For this review, take the finished solid that the model builds, in its own axes (mm). Round coordinates to 2 decimals unless told otherwise and drop trailing zeros. Order: outer loops, then holes, each group sorted by start corner. A loop starts at its lowest first (then second) coordinate and runs counter-clockwise, first axis right, second up. Notation, with made-up numbers: (2.25, 31.5) -> (36.25, 31.5) arc R15 ccw to (36.25, 39.5) -> close; hole circle Ø5 at (42.5, 54). An arc over 180 degrees is marked (long way). Use a Markdown table: item, result. Add a question column.
1) Wall thickness on line 1 along Z through (x, y) = (-2, -10.5); line 2 along X through (y, z) = (6.25, 0.5); line 3 along Y through (x, z) = (-40, 3.75): over which ranges is each line inside the solid? List them lowest first. Write a range as [from, to].
2) Clearance check with flat-ended pins moving along their axes: P1, Ø1.5, axis at y = 8, z = 0.5, coming from the -X side; P2, Ø1.1, axis at y = -14.5, z = -0.5, coming from the +X side; P3, Ø0.5, axis at x = 13, y = -14.5, coming from the +Z side; P4, Ø6.5, axis at x = -22, z = 0.5, coming from the -Y side. State where each tip first meets the part, or that it passes through.
3) Consider section B-B (x = -285.5). State the section outline as (y, z) points, plus the area to 3 significant figures.
4) Consider section A-A (x = 14.5). State the section outline as (y, z) points.
```python
from build123d import *

# Parameters (mm, degrees)
SKETCH_W        = 100
SKETCH_H        = 30
PAD_DEPTH       = 5.5
FILLET_R        = 5
THICKNESS_T     = -1
PAD001_DEPTH    = 2
CHAMFER_SIZE    = 1
SKETCH002_R     = 3
HOLE_DEPTH      = 25
HOLE_TIPS_R     = 3
SKETCH003_R     = 0.75
SKETCH003_W     = 14
SKETCH003_H     = 6
POCKET_DEPTH    = 5
SKETCH004_R     = 3.25
PAD002_DEPTH    = 10
SKETCH005_R     = 2
PAD003_DEPTH    = 258.5
SKETCH006_R     = 2.5
PAD004_DEPTH    = 6
PAD005_DEPTH    = 18
PAD006_DEPTH    = 7.5
POCKET001_DEPTH = 7


with BuildPart() as part:
    # Sketch → Pad (new body, symmetric)
    with BuildSketch(Plane.XY):
        Rectangle(SKETCH_W, SKETCH_H)
    extrude(amount=PAD_DEPTH, both=True)

    # Fillet
    fillet_edges = [part.edges().sort_by_distance(p)[0] for p in [
        (-50, -15, 0),
        (-50, 15, 0),
        (50, 15, 0),
        (50, -15, 0),
    ]]
    fillet(fillet_edges, radius=FILLET_R)

    # Thickness
    thickness_openings = [part.faces().sort_by_distance(p)[0] for p in [
        (0, 0, -5.5),
    ]]
    offset(amount=THICKNESS_T, openings=thickness_openings)

    # Sketch001 (on Face10 of Thickness) → Pad001 (join)
    with BuildSketch(Plane(origin=(0, 0, -5.5), x_dir=(1, 0, 0), z_dir=(0, 0, -1))):
        with BuildLine():
            ThreePointArc((-45, 14), (-47.828427, 12.828427), (-49, 10))
            Line((-49, -10), (-49, 10))
            ThreePointArc((-49, -10), (-47.828427, -12.828427), (-45, -14))
            Line((45, -14), (-45, -14))
            ThreePointArc((45, -14), (47.828427, -12.828427), (49, -10))
            Line((49, 10), (49, -10))
            ThreePointArc((49, 10), (47.828427, 12.828427), (45, 14))
            Line((-45, 14), (45, 14))
        make_face()
    extrude(amount=-PAD001_DEPTH)

    # Chamfer
    chamfer_edges = [part.edges().sort_by_distance(p)[0] for p in [
        (0, -15, 5.5),
        (48.535534, -13.535534, 5.5),
        (50, 0, 5.5),
        (48.535534, 13.535534, 5.5),
        (0, 15, 5.5),
        (-48.535534, 13.535534, 5.5),
        (-50, 0, 5.5),
        (-48.535534, -13.535534, 5.5),
    ]]
    chamfer(chamfer_edges, length=CHAMFER_SIZE)

    # Sketch002 (on Face7 of Chamfer) → Hole (cut)
    with BuildSketch(Plane(origin=(-50, 0, 0), x_dir=(0, -1, 0), z_dir=(-1, 0, 0))):
        Circle(SKETCH002_R)
    extrude(amount=-HOLE_DEPTH, mode=Mode.SUBTRACT)

    # Hole tips → Hole tip 1 section 0
    with BuildSketch(Plane(origin=(-25, 0, 0), x_dir=(0, -1, 0), z_dir=(-1, 0, 0)), mode=Mode.PRIVATE) as hole_tip_1_s0:
        Circle(HOLE_TIPS_R)
    loft([hole_tip_1_s0.sketch, Vertex(-23.197418, 0, 0)], mode=Mode.SUBTRACT)

    # Sketch003 (on Face11 of Hole) → Pocket (cut)
    with BuildSketch(Plane.XZ.offset(15)):
        with Locations((-37.906574, 2.290524)):
            Circle(SKETCH003_R)
        with Locations((35.604452, 0)):
            Rectangle(SKETCH003_W, SKETCH003_H)
        with Locations((14.604452, 0)):
            Rectangle(SKETCH003_W, SKETCH003_H)
        with Locations((-6.395548, 0)):
            Rectangle(SKETCH003_W, SKETCH003_H)
        with Locations((-27.395548, 0)):
            Rectangle(SKETCH003_W, SKETCH003_H)
    extrude(amount=-POCKET_DEPTH, mode=Mode.SUBTRACT)

    # Sketch004 (on Face7 of Pocket) → Pad002 (join)
    with BuildSketch(Plane(origin=(-50, 0, 0), x_dir=(0, -1, 0), z_dir=(-1, 0, 0))):
        Circle(SKETCH004_R)
    extrude(amount=PAD002_DEPTH)

    # Sketch005 (on Face38 of Pad002) → Pad003 (join)
    with BuildSketch(Plane(origin=(-60, 0, 0), x_dir=(0, -1, 0), z_dir=(-1, 0, 0))):
        Circle(SKETCH005_R)
    extrude(amount=PAD003_DEPTH)

    # Sketch006 (on Face45 of Pad003) → Pad004 (join)
    with BuildSketch(Plane(origin=(-318.5, 0, 0), x_dir=(0, -1, 0), z_dir=(-1, 0, 0))):
        Circle(SKETCH006_R)
    extrude(amount=PAD004_DEPTH)

    # Sketch007 (on Face3 of Pad004) → Pad005 (join)
    with BuildSketch(Plane(origin=(-324.5, 0, 0), x_dir=(0, -1, 0), z_dir=(-1, 0, 0))):
        with BuildLine():
            ThreePointArc((-3, 2.5), (-5.5, 0), (-3, -2.5))
            Line((-3, -2.5), (3, -2.5))
            ThreePointArc((3, -2.5), (5.5, 0), (3, 2.5))
            Line((3, 2.5), (-3, 2.5))
        make_face()
    extrude(amount=PAD005_DEPTH)

    # Sketch008 (on Face11 of Pad005) → Pad006 (join)
    with BuildSketch(Plane(origin=(-342.5, 0, 0), x_dir=(0, -1, 0), z_dir=(-1, 0, 0))):
        with BuildLine():
            ThreePointArc((-3.25, 1.25), (-4.5, 0), (-3.25, -1.25))
            Line((-3.25, -1.25), (3.25, -1.25))
            ThreePointArc((3.25, -1.25), (4.5, 0), (3.25, 1.25))
            Line((3.25, 1.25), (-3.25, 1.25))
        make_face()
    extrude(amount=PAD006_DEPTH)

    # Sketch009 (on Face18 of Pad006) → Pocket001 (cut)
    with BuildSketch(Plane(origin=(-350, 0, 0), x_dir=(0, -1, 0), z_dir=(-1, 0, 0))):
        with BuildLine():
            ThreePointArc((-3.288859, 0.763778), (-4.052637, 0), (-3.288859, -0.763778))
            Line((-3.288859, -0.763778), (3.288859, -0.763778))
            ThreePointArc((3.288859, -0.763778), (4.052637, 0), (3.288859, 0.763778))
            Line((3.288859, 0.763778), (-3.288859, 0.763778))
        make_face()
    extrude(amount=-POCKET001_DEPTH, mode=Mode.SUBTRACT)


solid = part.part
```
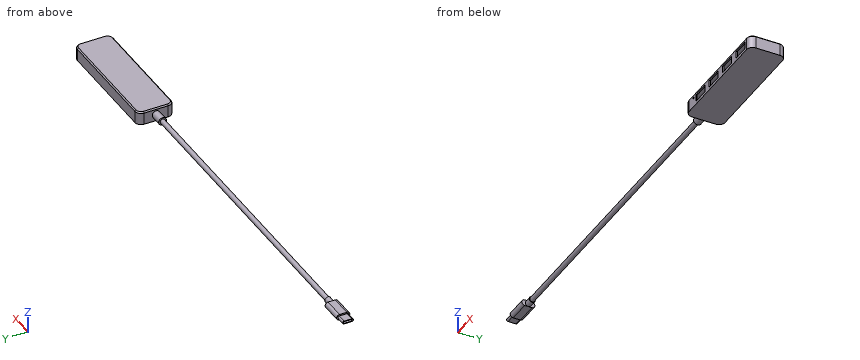
Results list:
| question | item | result |
|---|---|---|
| 1 | line 1 | [-5.5, -3.5], [4.5, 5.5] |
| 1 | line 2 | [-50, -49], [49, 50] |
| 1 | line 3 | [-15, -14], [14, 15] |
| 2 | P1 | x = -50 |
| 2 | P2 | x = 48.07 |
| 2 | P3 | z = 5.25 |
| 2 | P4 | y = -15 |
| 3 | outline | circle Ø4 at (0, 0) |
| 3 | area | 12.6 mm2 |
| 4 | outline | (-15, -5.5) -> (15, -5.5) -> (15, 4.5) -> (14, 5.5) -> (-14, 5.5) -> (-15, 4.5) -> (-15, 3) -> (-14, 3) -> (-14, 4.5) -> (14, 4.5) -> (14, -3.5) -> (-14, -3.5) -> (-14, -3) -> (-15, -3) -> close |
